```python
from build123d import *

# Parameters (mm, degrees)
ANGLE_IRON_35_X_35_X_5_1_DEPTH = 65


with BuildPart() as part:
    # Sketch11 → Angle iron 35 X 35 X 5(1) (new body)
    with BuildSketch(Plane.YZ.offset(-32.229166667)):
        with BuildLine():
            Line((0, 0), (0, 35))
            ThreePointArc((0, 35), (3.535533906, 33.535533906), (5, 30))
            Line((5, 30), (5, 10))
            ThreePointArc((5, 10), (6.464466094, 6.464466094), (10, 5))
            Line((10, 5), (30, 5))
            ThreePointArc((30, 5), (33.535533906, 3.535533906), (35, 0))
            Line((35, 0), (0, 0))
        make_face()
    extrude(amount=ANGLE_IRON_35_X_35_X_5_1_DEPTH)


solid = part.part
```
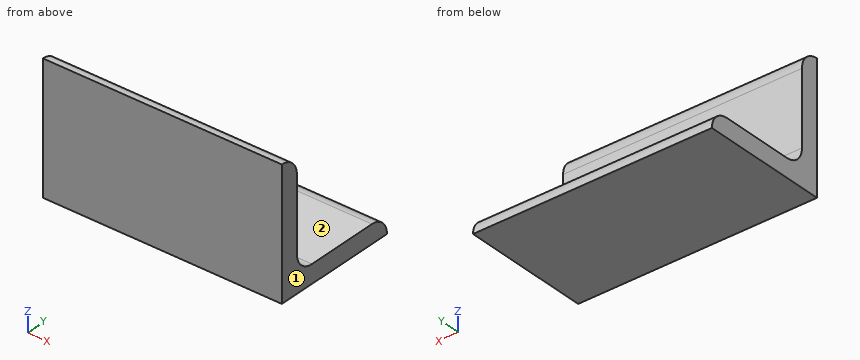
Check sheet for the modelled part. Datum: model origin and axes. Units: mm. Face numbers are marked on the shaded views. A direction names the side the tool comes from. Give positions to 0.01 mm unless a question says otherwise; leave off trailing zeros. Order: outer loops, then holes, each group sorted by start corner. A loop starts at its lowest first (then second) coordinate and runs counter-clockwise, first axis right, second up. Notation, with made-up numbers: (-36.5, 62.5) -> (-30.5, 62.5) arc R16 cw to (-30.5, 82.5) -> close; hole circle Ø1 at (10.25, -10.75). An arc over 180 degrees is marked (long way). Use CSV: the item, a comma, the result in double quotes. Start each with the question number.
1) Go/stop test with flat-tipped pins: P1, Ø12, axis at x = 0, z = 23, coming from the -Y side; P2, Ø2, axis at x = -12, z = 22, coming from the +Y side. Record where each tip stops, or that it passes through.
2) Sectioned sample at B-B, the plane y = 23. Record the boundary of the cut face in (x, z).
3) Set-up check for the marked faces 1 and 2: record each of +Z, -Z, +X, -X, +Y, -Y from which the full face is reachable in a straight line by a thin tool's end or side.
4) Material ranges on line 1 (Z direction, x = 5, y = 20); line 2 (Z direction, x = 19.5, y = 33.5), recorded low to high. Write a range as from..to.
5) Sectioned sample at C-C, the plane z = 4. Record the boundary of the cut face in (x, y), plus the area to 4 significant figures.
6) Sectioned sample at A-A, the plane x = -17. Record the boundary of the cut face in (y, z), plus the area to 3 significant figures.
Recorded:
1,P1,"y = 0"
1,P2,"y = 5"
2,outline,"(-32.23, 0) -> (32.77, 0) -> (32.77, 5) -> (-32.23, 5) -> close"
3,face 1,"+Z, -Z, +X, +Y, -Y"
3,face 2,"+Z, +X, -X, +Y"
4,line 1,"0..5"
4,line 2,"0..3.57"
5,outline,"(-32.23, 0) -> (32.77, 0) -> (32.77, 33) -> (-32.23, 33) -> close"
5,area,"2,145 mm2"
6,outline,"(0, 0) -> (35, 0) arc R5 ccw to (30, 5) -> (10, 5) arc R5 cw to (5, 10) -> (5, 30) arc R5 ccw to (0, 35) -> close"
6,area,"320 mm2"
